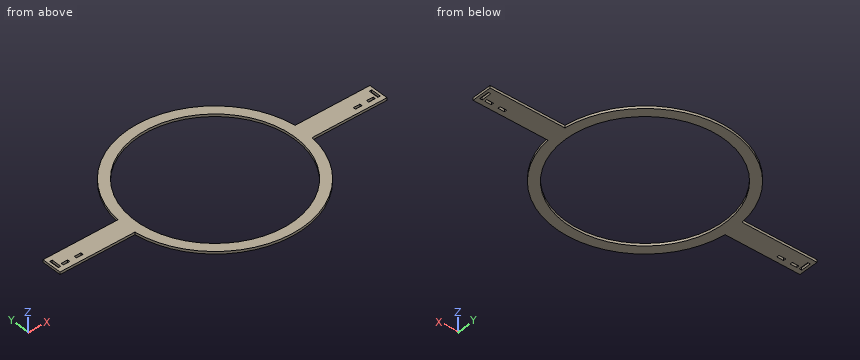
from build123d import *

# Parameters (mm, degrees)
SKETCH1_R           = 114.3
SKETCH1_R_2         = 101.6
BOSS_EXTRUDE1_DEPTH = 3.175
SKETCH2_W           = 3.175
SKETCH2_H           = 12.7
CUT_EXTRUDE1_DEPTH  = 3.175
SKETCH3_W           = 8.466666667
SKETCH3_H           = 3.175
CUT_EXTRUDE2_DEPTH  = 3.175


with BuildPart() as part:
    # Sketch1 → Boss-Extrude1 (new body)
    # profile 1 of 3: a face of its own
    with BuildSketch(Plane.XY):
        with BuildLine():
            Line((-209.55, -12.7), (-113.592253257, -12.7))
            ThreePointArc((-113.592253257, -12.7), (-114.3, 0), (-113.592253257, 12.7))
            Line((-113.592253257, 12.7), (-209.55, 12.7))
            Line((-209.55, 12.7), (-209.55, -12.7))
        make_face()
    # profile 2 of 3: a face of its own
    with BuildSketch(Plane.XY):
        Circle(SKETCH1_R)
        Circle(SKETCH1_R_2, mode=Mode.SUBTRACT)
    # profile 3 of 3: a face of its own
    with BuildSketch(Plane.XY):
        with BuildLine():
            ThreePointArc((114.3, 0), (114.122926153, -6.3598527), (113.592253257, -12.7))
            Line((113.592253257, -12.7), (209.55, -12.7))
            Line((209.55, -12.7), (209.55, 12.7))
            Line((209.55, 12.7), (113.592253257, 12.7))
            ThreePointArc((113.592253257, 12.7), (114.122926153, 6.3598527), (114.3, 0))
        make_face()
    extrude(amount=BOSS_EXTRUDE1_DEPTH)

    # Sketch2 → Cut-Extrude1 (cut)
    with BuildSketch(Plane.XY.offset(3.175)):
        with Locations((-204.7875, 0)):
            Rectangle(SKETCH2_W, SKETCH2_H)
    cut_extrude1 = extrude(amount=-CUT_EXTRUDE1_DEPTH, mode=Mode.SUBTRACT)

    # Mirror1: Cut-Extrude1 across plane
    add(cut_extrude1.mirror(Plane(origin=(0, 0, 0), x_dir=(0, 0, 1), z_dir=(1, 0, 0))), mode=Mode.SUBTRACT)

    # Sketch3 → Cut-Extrude2 (cut)
    with BuildSketch(Plane.XY.offset(3.175)):
        with Locations((195.791666667, -4.7625)):
            Rectangle(SKETCH3_W, SKETCH3_H)
        with Locations((178.858333334, -4.7625)):
            Rectangle(SKETCH3_W, SKETCH3_H)
    cut_extrude2 = extrude(amount=-CUT_EXTRUDE2_DEPTH, mode=Mode.SUBTRACT)

    # Mirror2: Cut-Extrude2 across plane
    add(cut_extrude2.mirror(Plane(origin=(0, 0, 0), x_dir=(0, 0, 1), z_dir=(1, 0, 0))), mode=Mode.SUBTRACT)


solid = part.part
Work out the finished part from the listing and answer in its coordinate system (mm). Coordinates: 2 decimals unless noted, no trailing zeros. Write each loop counter-clockwise with the first axis right and the second up, starting at its lowest first coordinate (ties: lowest second). Pieces come first, ordered by that corner, then holes. Notation, with made-up numbers: M -18.75,29.5 L 32.25,29.5 A23 ccw 32.25,41.5 Z; hole C -30,31.25 d5. An arc over 180 degrees is marked long. Use one line per item in the form item = value. Start each with the question number.
1. The part is cut by section C-C (z = 0.75). Give the number of separate pieces and of enclosed holes in the cut face, plus the area to 3 significant figures.
2. Each of these flat-tipped pins is pushed along its axis until it touches: P1, Ø1, axis at x = 204, z = 1.5, coming from the -Y side; P2, Ø1, axis at y = 34, z = 2, coming from the -X side; P3, Ø1, axis at x = -197.5, z = 1, coming from the +Y side; P4, Ø8, axis at x = -96.5, y = -71, coming from the +Z side. Where does it stop, or does it pass through?
3. The part is cut by section B-B (y = -84.5). Give the vertices of the cut face in (x, z) (3 decimals), plus the area to 3 significant figures.
4. Straight lines are drawn through the part: probe 1 along Y at (x, z) = (0, 2.25); probe 2 along Y at (x, z) = (-145, 2.65); probe 3 along Y at (x, z) = (8, 2.6). For each, find the intervals that lie inside material, in ascending order. Write a range as from..to.
5. The part is cut by section A-A (x = 0). Give the vertices of the cut face in (y, z) (3 decimals).
Evaluation:
q1.separate_pieces = 1
q1.enclosed_holes = 7
q1.area = 13,300 mm^2
q2.P1 = -12.7
q2.P2 = -109.28
q2.P3 = 12.7
q2.P4 = through
q3.outline = M -76.969,0 L -56.412,0 L -56.412,3.175 L -76.969,3.175 Z; M 56.412,0 L 76.969,0 L 76.969,3.175 L 56.412,3.175 Z
q3.area = 131 mm^2
q4.probe_1 = -114.3..-101.6, 101.6..114.3
q4.probe_2 = -12.7..12.7
q4.probe_3 = -114.02..-101.28, 101.28..114.02
q5.outline = M -114.3,0 L -101.6,0 L -101.6,3.175 L -114.3,3.175 Z; M 101.6,0 L 114.3,0 L 114.3,3.175 L 101.6,3.175 Z
